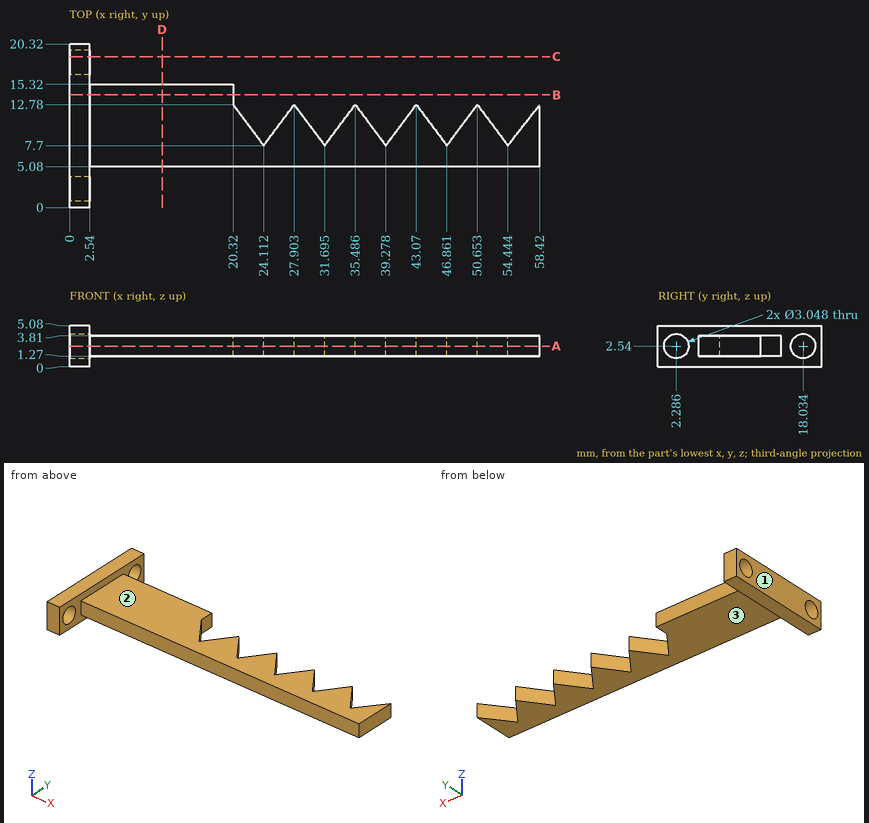
For this review, use the dimensioned drawing (mm, ordinates from the lowest corner) and the shaded views. A direction names the side the tool comes from. Coordinates: 2 decimals unless noted, no trailing zeros. Order: outer loops, then holes, each group sorted by start corner. A loop starts at its lowest first (then second) coordinate and runs counter-clockwise, first axis right, second up. Notation, with made-up numbers: (51.5, 25) - (72.5, 25) arc R25 ccw to (72.5, 63) - close; hole circle Ø6 at (25.25, -33.5). An arc over 180 degrees is marked (long way). Answer in a Markdown table with one row per item.
(1) Wall thickness on line 1 along Y through (x, z) = (0.7, 2.54); line 2 along X through (y, z) = (10, 3.75) (1 decimal); line 3 along Z through (x, y) = (12, 13.75): over which ranges is each line inside the solid? List them lowest first. Write a range as from..to.
Checked values:
| item | result |
|---|---|
| line 1 | 0..0.76, 3.81..16.51, 19.56..20.32 |
| line 2 | 0..22.4, 25.8..30, 33.4..37.6, 41..45.1, 48.6..52.7, 56.2..58.4 |
| line 3 | 1.27..3.81 |
(2) Consider section C-C on y = 18.75. State the section outline as (x, z) points (1 decimal).
Checked values:
| item | result |
|---|---|
| outline | (0, 0) - (2.5, 0) - (2.5, 1.2) - (0, 1.2) - close; (0, 3.9) - (2.5, 3.9) - (2.5, 5.1) - (0, 5.1) - close |
(3) Clearance check with flat-ended pins moving along their axes: pin 1 (3 mm diameter, centred on x = 14, z = 3.5, fed in from -Y); pin 2 (3 mm diameter, centred on x = 17.5, y = 11.5, fed in from +Z); pin 3 (11.5 mm diameter, centred on x = 21, y = 11.5, fed in from -Z); pin 4 (2.5 mm diameter, centred on y = 2.286, z = 2.54, fed in from +X). State where each tip first meets the part, or that it passes through.
Checked values:
| item | result |
|---|---|
| pin 1 | y = 5.08 |
| pin 2 | z = 3.81 |
| pin 3 | z = 1.27 |
| pin 4 | through |
(4) Consider section B-B on y = 14. State the section outline as (x, z) points.
Checked values:
| item | result |
|---|---|
| outline | (0, 0) - (2.54, 0) - (2.54, 1.27) - (20.32, 1.27) - (20.32, 3.81) - (2.54, 3.81) - (2.54, 5.08) - (0, 5.08) - close |
(5) Consider section A-A on z = 2.54. State the section outline as (x, y) points (1 decimal), plus the area to 3 significant figures.
Checked values:
| item | result |
|---|---|
| outline | (0, 0) - (2.5, 0) - (2.5, 0.8) - (0, 0.8) - close; (0, 3.8) - (2.5, 3.8) - (2.5, 5.1) - (58.4, 5.1) - (58.4, 12.8) - (54.4, 7.7) - (50.7, 12.8) - (46.9, 7.7) - (43.1, 12.8) - (39.3, 7.7) - (35.5, 12.8) - (31.7, 7.7) - (27.9, 12.8) - (24.1, 7.7) - (20.3, 12.8) - (20.3, 15.3) - (2.5, 15.3) - (2.5, 16.5) - (0, 16.5) - close; (0, 19.6) - (2.5, 19.6) - (2.5, 20.3) - (0, 20.3) - close |
| area | 415 mm^2 |
(6) Consider section D-D on x = 11.5. State the section outline as (y, z) points, plus the area to 3 significant figures.
Checked values:
| item | result |
|---|---|
| outline | (5.08, 1.27) - (15.32, 1.27) - (15.32, 3.81) - (5.08, 3.81) - close |
| area | 26.0 mm^2 |
(7) For the marked faces 1, 2 and 3, list the 3-axis set-ups (+Z, -Z, +X, -X, +Y, -Y) from which the entire face can be reached by the end or side of a thin tool; tool diameter is ignored.
Checked values:
| item | result |
|---|---|
| face 1 | +Z, -Z, -X, +Y, -Y |
| face 2 | +Z, +X, +Y, -Y |
| face 3 | -Z, +X, +Y, -Y |
